Autodesk Inventor part; units mm, degrees
ref_plane "YZ Plane" through (0, 0, 0) normal (1, 0, 0) x (0, 1, 0)
ref_plane "XZ Plane" through (0, 0, 0) normal (0, 1, 0) x (-1, 0, 0)
ref_plane "XY Plane" through (0, 0, 0) normal (0, 0, 1) x (1, 0, 0)
sketch "Sketch1" plane through (0, 0, 0) normal (0, 0, 1) x (1, 0, 0)
  circle A0 centre (0, 0) radius 12.7
  circle A1 centre (0, 0) radius 12.446
  circle A2 centre (0, 0) radius 6.35
  circle A3 centre (0, 0) radius 5.8601
  dimension "d1" = 25.4
  dimension "d2" = 24.892
  dimension "d3" = 12.7
extrude "Extrusion1" [suppressed]
extrude "Extrusion2" add sketch "Sketch1" along normal blind 6.858 and the other way blind 6.858 contours A0
extrude "Extrusion3" add sketch "Sketch1" along normal blind 2.54 and the other way blind 2.54 contours A1
extrude "Extrusion4" add sketch "Sketch1" along normal blind 6.35 and the other way blind 6.35 contours A2
fillet "Fillet1" [suppressed]
properties part number "plastic idler wheel base part"
CAD build for the part. Positions are in the model's coordinates, mm. A direction names the side the tool comes from. Give positions to 0.01 mm unless a question says otherwise; leave off trailing zeros. Order: outer loops, then holes, each group sorted by start corner. A loop starts at its lowest first (then second) coordinate and runs counter-clockwise, first axis right, second up. Notation, with made-up numbers: M -16.75,21 L -11.75,21 A19 ccw -11.75,49 Z; hole C 41.5,85.25 d11. An arc over 180 degrees is marked long. Put each result on its own line as item: value. Start each with the question number.
(1) Saw through at A-A, the plane x = 0. Write the cut outline in (y, z), then the cut area to 3 significant figures.
(2) Mould opens along Y. For faces 1 (the cylindrical face through (-1.38, 6.2, 4.42)), 2 (the cylindrical face through (-2.75, -12.4, 0.1)) say: +Y half, -Y half, draft (parallel to the pull), parting line (faces both ways), or undercut.
(3) Saw through at C-C, the plane z = 5.25. Write the cut outline in (x, y), then the cut area to 3 significant figures.
(4) Saw through at D-D, the plane z = 0.5. Write the cut outline in (x, y), then the cut area to 3 significant figures.
(5) Saw through at B-B, the plane y = 2. Write the cut outline in (x, z).
(6) Flat gauge pins, fed straight in: pin 1 Ø1 at (x, z) = (-7.5, -4) entering from -Y; pin 2 Ø15 at (x, y) = (0, 0) entering from -Z; pin 3 Ø10 at (x, y) = (1, -3) entering from +Z; pin 4 Ø5 at (x, y) = (2.5, 1.5) entering from +Z. Where does each tip first touch, or does it go through?
(7) Which spindle directions (+Z, -Z, +X, -X, +Y, -Y) get a long thin tool onto all of the face, cutting with end or side? Do faces 3 (the cylindrical face through (-1.38, -6.2, -4.42)), 4 (the cylindrical face through (-2.7, 12.15, 4.67)), 5 (the cylindrical face through (3.15, -4.94, -0.09)). Say none if no direction does.
(8) Drill centre lines: line 1 along Y through (x, z) = (0, 4.3); line 2 along X through (y, z) = (-1, -3.5); line 3 along X through (y, z) = (1.25, 4). Where is each one in solid material? Low to high.
Check result:
1. outline: M -12.7,-6.86 L -12.45,-6.86 L -12.45,-2.54 L -6.35,-2.54 L -6.35,-6.35 L -5.86,-6.35 L -5.86,6.35 L -6.35,6.35 L -6.35,2.54 L -12.45,2.54 L -12.45,6.86 L -12.7,6.86 Z; M 5.86,-6.35 L 6.35,-6.35 L 6.35,-2.54 L 12.45,-2.54 L 12.45,-6.86 L 12.7,-6.86 L 12.7,6.86 L 12.45,6.86 L 12.45,2.54 L 6.35,2.54 L 6.35,6.35 L 5.86,6.35 Z
1. area: 81.3 mm2
2. face 1: undercut
2. face 2: parting line
3. outline: C 0,0 d25.4; C 0,0 d12.7; hole C 0,0 d24.89; hole C 0,0 d11.72
3. area: 38.9 mm2
4. outline: C 0,0 d25.4; hole C 0,0 d11.72
4. area: 399 mm2
5. outline: M -12.54,-6.86 L -12.28,-6.86 L -12.28,-2.54 L -6.03,-2.54 L -6.03,-6.35 L -5.51,-6.35 L -5.51,6.35 L -6.03,6.35 L -6.03,2.54 L -12.28,2.54 L -12.28,6.86 L -12.54,6.86 Z; M 5.51,-6.35 L 6.03,-6.35 L 6.03,-2.54 L 12.28,-2.54 L 12.28,-6.86 L 12.54,-6.86 L 12.54,6.86 L 12.28,6.86 L 12.28,2.54 L 6.03,2.54 L 6.03,6.35 L 5.51,6.35 Z
6. pin 1: stops at y = -10.6
6. pin 2: stops at z = -6.35
6. pin 3: stops at z = 6.35
6. pin 4: passes through
7. face 3: -Z
7. face 4: +Z
7. face 5: +Z, -Z
8. line 1: y = -12.7 to -12.45, -6.35 to -5.86, 5.86 to 6.35, 12.45 to 12.7
8. line 2: x = -12.66 to -12.41, -6.27 to -5.77, 5.77 to 6.27, 12.41 to 12.66
8. line 3: x = -12.64 to -12.38, -6.23 to -5.73, 5.73 to 6.23, 12.38 to 12.64
